Can you work these out from the model? Positions are in its coordinate system, mm. Give positions to 0.01 mm unless a question says otherwise; leave off trailing zeros. Loops run counter-clockwise (first coordinate to the right, second up) from the corner with the lowest first, then second, coordinate; pieces in that order, holes last. Notation, with made-up numbers: M -14,69.5 L 36,69.5 A26 cw 36,83.5 Z; hole C 75.25,9 d2. An arc over 180 degrees is marked long. Answer as a JSON object with one key per item and string values.
```python
from build123d import *

# Parameters (mm, degrees)
SKETCH1_R           = 2.1
BOSS_EXTRUDE1_DEPTH = 5


with BuildPart() as part:
    # Sketch1 → Boss-Extrude1 (new body)
    with BuildSketch(Plane.XY):
        with BuildLine():
            Line((51.628885754, 99.200000001), (300.816905308, 99.200000001))
            ThreePointArc((300.816905308, 99.200000001), (318.316905308, 81.700000001), (300.816905308, 64.200000001))
            Line((300.816905308, 64.200000001), (51.628885754, 64.200000001))
            ThreePointArc((51.628885754, 64.200000001), (34.128885754, 81.700000001), (51.628885754, 99.200000001))
        make_face()
        with Locations((300.816905308, 81.700000001)):
            Circle(SKETCH1_R, mode=Mode.SUBTRACT)
        with Locations((270.816905308, 81.700000001)):
            Circle(SKETCH1_R, mode=Mode.SUBTRACT)
        with Locations((191.222895531, 81.700000001)):
            Circle(SKETCH1_R, mode=Mode.SUBTRACT)
        with Locations((51.628885754, 81.700000001)):
            Circle(SKETCH1_R, mode=Mode.SUBTRACT)
        with Locations((81.628885754, 81.700000001)):
            Circle(SKETCH1_R, mode=Mode.SUBTRACT)
        with Locations((161.222895531, 81.700000001)):
            Circle(SKETCH1_R, mode=Mode.SUBTRACT)
    extrude(amount=BOSS_EXTRUDE1_DEPTH)


solid = part.part
```
1) Suppose I cut it at B-B, the plane y = 92. Write out the boundary of the cut face in (x, z), and give its area (3 significant figures).
Answer list:
{"outline": "M 37.48,0 L 314.96,0 L 314.96,5 L 37.48,5 Z", "area": "1,390 mm^2"}
2) Suppose I cut it at C-C, the plane y = 70. Write out the boundary of the cut face in (x, z), and give its area (3 significant figures).
Answer list:
{"outline": "M 38.62,0 L 313.83,0 L 313.83,5 L 38.62,5 Z", "area": "1,380 mm^2"}
3) Please list where these lines run through material, in increasing order: line 1 along X through (y, z) = (69, 3.5); line 2 along X through (y, z) = (88, 2.7); line 3 along Y through (x, z) = (83, 4.55). Write a range as from..to.
Answer list:
{"line 1": "39.59..312.86", "line 2": "35.3..317.14", "line 3": "64.2..80.11, 83.29..99.2"}
4) Will this pin go through, and if not, where does the flat tip stop? pin 1 Ø1 at (y, z) = (74.5, 2) entering from +X.
Answer list:
{"pin 1": "x = 316.98"}
5) Suppose I cut it at A-A, the plane z = 3.7. Write out the boundary of the cut face in (x, y).
Answer list:
{"outline": "M 51.63,64.2 L 300.82,64.2 A17.5 ccw 300.82,99.2 L 51.63,99.2 A17.5 ccw Z; hole C 51.63,81.7 d4.2; hole C 81.63,81.7 d4.2; hole C 161.22,81.7 d4.2; hole C 191.22,81.7 d4.2; hole C 270.82,81.7 d4.2; hole C 300.82,81.7 d4.2"}
